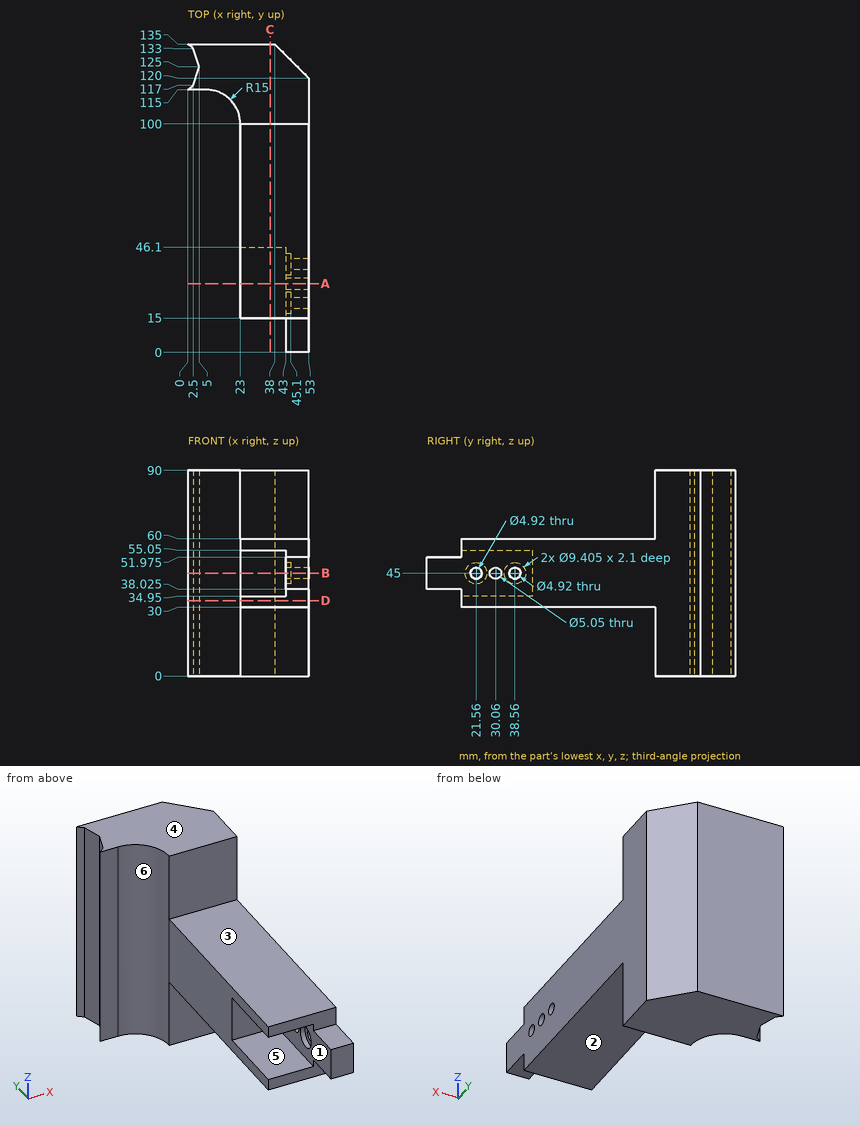
Part print with two shaded views. Sizes in mm from the minimum x, y, z corner. A direction names the side the tool comes from. Round coordinates to 2 decimals unless told otherwise and drop trailing zeros. Order: outer loops, then holes, each group sorted by start corner. A loop starts at its lowest first (then second) coordinate and runs counter-clockwise, first axis right, second up. Notation, with made-up numbers: (65.25, 63) - (76.25, 63) arc R18 cw to (76.25, 98) - close; hole circle Ø11 at (41.25, 61.25). An arc over 180 degrees is marked (long way). Return JSON: item names as keys, results as strings.
(1) Cut at C-C (x = 36). Give the cut face in (y, z), then the cut area to 3 significant figures.
Answer key:
{"outline": "(15, 30) - (100, 30) - (100, 0) - (135, 0) - (135, 90) - (100, 90) - (100, 60) - (15, 60) - (15, 55.05) - (46.1, 55.05) - (46.1, 34.95) - (15, 34.95) - close", "area": "5,070 mm^2"}
(2) Cut at B-B (z = 45). State how many separate pieces and enclosed holes the cut face has, then the cut area to 3 significant figures.
Answer key:
{"separate pieces": "4", "enclosed holes": "0", "area": "3,290 mm^2"}
(3) Tool access for the marked faces 1, 2 and 3: list every direction of +Z, -Z, +X, -X, +Y, -Y with a clear straight run to the whole face (end or side of a thin tool).
Answer key:
{"face 1": "-X, -Y", "face 2": "-Z, +X, -X, -Y", "face 3": "+Z, +X, -X, -Y"}
(4) Pin check, flat tips, straight feed: pin 1 Ø6.5 at (x, z) = (5, 50.5) entering from -Y; pin 2 Ø10 at (x, y) = (47, 87) entering from -Z; pin 3 Ø10 at (x, y) = (15, 18) entering from +Z; pin 4 Ø3 at (x, y) = (47.5, 8) entering from +Z (3 decimals). Stop position of each tip, or through.
Answer key:
{"pin 1": "stops at y = 115", "pin 2": "stops at z = 30", "pin 3": "passes through", "pin 4": "stops at z = 51.975"}
(5) Wall check: probe 1 along Z at (x, y) = (48.5, 38.56); probe 2 along Y at (x, z) = (49, 45) (3 decimals); probe 3 along Y at (x, z) = (48.5, 45) (3 decimals). Give the ranges that are in metal, low to high. Write a range as from..to.
Answer key:
{"probe 1": "z = 30..42.54, 47.46..60", "probe 2": "y = 0..19.1, 24.02..27.535, 32.585..36.1, 41.02..124", "probe 3": "y = 0..19.1, 24.02..27.535, 32.585..36.1, 41.02..124.5"}
(6) Pull direction Z, two halves, no side cores. Call the marked faces 4, 5 and 6: +Z half, -Z half, draft (parallel to the pull), parting line (faces both ways), or undercut.
Answer key:
{"face 4": "+Z half", "face 5": "undercut", "face 6": "draft"}
(7) Cut at D-D (z = 33). Give the cut face in (x, y).
Answer key:
{"outline": "(0, 115) - (8, 115) arc R15 cw to (23, 100) - (23, 15) - (53, 15) - (53, 120) - (38, 135) - (0, 135) - (2.5, 133) - (5, 125) - (2.5, 117) - close"}
(8) Cut at A-A (y = 30.06). Give the cut face in (x, z) (3 decimals).
Answer key:
{"outline": "(23, 30) - (53, 30) - (53, 42.475) - (43, 42.475) - (43, 34.95) - (23, 34.95) - close; (23, 55.05) - (43, 55.05) - (43, 47.525) - (53, 47.525) - (53, 60) - (23, 60) - close"}
